```python
from build123d import *

# Parameters (mm, degrees)
CYLINDER030_R     = 1.6
CYLINDER030_DEPTH = 50
CYLINDER029_R     = 5
CYLINDER029_DEPTH = 22.5
CYLINDER031_R     = 1.6
CYLINDER031_DEPTH = 50
BOX019_W          = 35
BOX019_H          = 27
BOX019_DEPTH      = 3


with BuildPart() as cylinder030:
    # Cylinder030 → Cylinder030 (new body)
    with BuildSketch(Plane(origin=(20.4, 8.8, -22), x_dir=(1, 0, 0), z_dir=(0, 0, 1))):
        Circle(CYLINDER030_R)
    extrude(amount=CYLINDER030_DEPTH)


with BuildPart() as fusion034:
    # Cylinder029 → Cylinder029 (new body)
    with BuildSketch(Plane.XY.offset(-12)):
        Circle(CYLINDER029_R)
    extrude(amount=CYLINDER029_DEPTH)

    # Fusion034: union Cylinder030
    add(cylinder030.part)


with BuildPart() as motor_holes_y:
    # Cylinder031 → Cylinder031 (new body)
    with BuildSketch(Plane(origin=(20.4, -8.8, -22), x_dir=(1, 0, 0), z_dir=(0, 0, 1))):
        Circle(CYLINDER031_R)
    extrude(amount=CYLINDER031_DEPTH)

    # Fusion036: union Fusion034
    add(fusion034.part)


with BuildPart() as motor_spacer:
    # Box019 → Box019 (new body)
    with BuildSketch(Plane(origin=(-10, -13, 0), x_dir=(1, 0, 0), z_dir=(0, 0, 1))):
        with Locations((17.5, 13.5)):
            Rectangle(BOX019_W, BOX019_H)
    extrude(amount=BOX019_DEPTH)

    # Cut030: cut motor-holes-y
    add(motor_holes_y.part, mode=Mode.SUBTRACT)


solid = motor_spacer.part
```
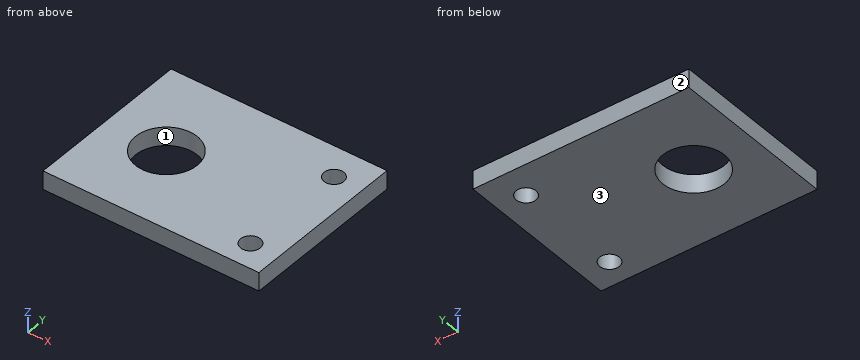
Model file for the job. Use its own axes, mm. Face numbers are marked on the shaded views. Coordinates: 2 decimals unless noted, no trailing zeros. Order: outer loops, then holes, each group sorted by start corner. A loop starts at its lowest first (then second) coordinate and runs counter-clockwise, first axis right, second up. Notation, with made-up numbers: (-38, -1.75) -> (-28, -1.75) arc R9 cw to (-28, 3.25) -> close; hole circle Ø4 at (36, -19). An arc over 180 degrees is marked (long way). Answer as a JSON object with one key per item and string values. Group by question number.
1) Cut at A-A, the plane x = -4. Write the cut outline in (y, z).
2) Cut at D-D, the plane z = 2.4. Write the cut outline in (x, y), then the cut area to 3 significant figures.
3) Cut at B-B, the plane x = 20.4. Write the cut outline in (y, z).
4) Pull direction Y, two halves, no side cores. Call the marked faces 1, 2 and 3: +Y half, -Y half, draft (parallel to the pull), parting line (faces both ways), or undercut.
5) Drill centre lines: L1, parallel to Y at x = 20.4, z = 1.65; L2, parallel to X at y = 0, z = 1.65; L3, parallel to X at y = 8.8, z = 2.3. Where is each one in solid material? Low to high.
6) Cut at C-C, the plane y = -8.8. Write the cut outline in (x, z), then the cut area to 3 significant figures.
Check values:
{
 "1": {"outline": "(-13, 0) -> (-3, 0) -> (-3, 3) -> (-13, 3) -> close; (3, 0) -> (14, 0) -> (14, 3) -> (3, 3) -> close"},
 "2": {"outline": "(-10, -13) -> (25, -13) -> (25, 14) -> (-10, 14) -> close; hole circle Ø10 at (0, 0); hole circle Ø3.2 at (20.4, -8.8); hole circle Ø3.2 at (20.4, 8.8)", "area": "850 mm²"},
 "3": {"outline": "(-13, 0) -> (-10.4, 0) -> (-10.4, 3) -> (-13, 3) -> close; (-7.2, 0) -> (7.2, 0) -> (7.2, 3) -> (-7.2, 3) -> close; (10.4, 0) -> (14, 0) -> (14, 3) -> (10.4, 3) -> close"},
 "4": {"face 1": "undercut", "face 2": "+Y half", "face 3": "draft"},
 "5": {"L1": "y = -13 to -10.4, -7.2 to 7.2, 10.4 to 14", "L2": "x = -10 to -5, 5 to 25", "L3": "x = -10 to 18.8, 22 to 25"},
 "6": {"outline": "(-10, 0) -> (18.8, 0) -> (18.8, 3) -> (-10, 3) -> close; (22, 0) -> (25, 0) -> (25, 3) -> (22, 3) -> close", "area": "95.4 mm²"}
}
